Work out the finished part from the listing and answer in its coordinate system (mm). A direction names the side the tool comes from. Round coordinates to 2 decimals unless told otherwise and drop trailing zeros. Write each loop counter-clockwise with the first axis right and the second up, starting at its lowest first coordinate (ties: lowest second). Pieces come first, ordered by that corner, then holes. Notation, with made-up numbers: (55, -7.75) - (89, -7.75) arc R6 ccw to (89, -3.75) - close; hole circle Ø5 at (15.5, 87). An arc over 180 degrees is marked (long way). Write item = value, one per line. Start each with the question number.
from build123d import *

# Parameters (mm, degrees)
F0_W      = 800.1
F0_H      = 533.4
F1_DEPTH  = 1492.25
F2_W      = 647.7
F2_H      = 200.025
F2_W_2    = 311.15
F2_H_2    = 863.6
F3_DEPTH  = 12.7
F2_H_3    = 50.8
F4_DEPTH  = 533.401
F5_W      = 368.3
F5_H      = 50.8
F6_DEPTH  = 800.101
F7_W      = 596.9
F7_H      = 317.5
F8_DEPTH  = 1371.6
F9_R      = 19.05
F10_DEPTH = 12.7


with BuildPart() as f1:
    # F0 (on Top) → F1 (new body)
    with BuildSketch(Plane.XY):
        Rectangle(F0_W, F0_H)
    extrude(amount=F1_DEPTH)

    # F2 (on face) → F3 (cut)
    with BuildSketch(Plane.XZ.offset(266.7)):
        Polygon((-400.05, 0), (-323.85, 0), (-323.85, 50.8), (323.85, 50.8), (323.85, 0), (400.05, 0), (400.05, 1466.85), (-400.05, 1466.85), align=None)
        with Locations((0, 201.6125)):
            Rectangle(F2_W, F2_H, mode=Mode.SUBTRACT)
        with Locations((0, 427.0375)):
            Rectangle(F2_W, F2_H, mode=Mode.SUBTRACT)
        with Locations((-168.275, 984.25)):
            Rectangle(F2_W_2, F2_H_2, mode=Mode.SUBTRACT)
        with Locations((168.275, 984.25)):
            Rectangle(F2_W_2, F2_H_2, mode=Mode.SUBTRACT)
    extrude(amount=-F3_DEPTH, mode=Mode.SUBTRACT)

    # F2 (on face) → F4 (cut, through all)
    with BuildSketch(Plane.XZ.offset(266.7)):
        with Locations((0, 25.4)):
            Rectangle(F2_W, F2_H_3)
    extrude(amount=-F4_DEPTH, mode=Mode.SUBTRACT)

    # F5 (on face) → F6 (cut, through all)
    with BuildSketch(Plane.YZ.offset(400.05)):
        with Locations((6.35, 25.4)):
            Rectangle(F5_W, F5_H)
    extrude(amount=-F6_DEPTH, mode=Mode.SUBTRACT)

    # F7 (on face) → F8 (cut)
    with BuildSketch(Plane(origin=(0, 0, 50.8), x_dir=(1, 0, 0), z_dir=(0, 0, -1))):
        with Locations((0, -6.35)):
            Rectangle(F7_W, F7_H)
    extrude(amount=-F8_DEPTH, mode=Mode.SUBTRACT)

    # F9 (on face) → F10 (join)
    with BuildSketch(Plane.XZ.offset(266.7)):
        with Locations((-88.9, 984.25)):
            Circle(F9_R)
        with Locations((88.9, 984.25)):
            Circle(F9_R)
        with Locations((168.275, 427.0375)):
            Circle(F9_R)
        with Locations((-168.275, 427.0375)):
            Circle(F9_R)
        with Locations((-168.275, 201.6125)):
            Circle(F9_R)
        with Locations((168.275, 201.6125)):
            Circle(F9_R)
    extrude(amount=F10_DEPTH)


solid = f1.part
1. Each of these flat-tipped pins is pushed along its axis until it touches: pin 1 (10 mm diameter, centred on x = -71, y = -263, fed in from -Z); pin 2 (6.5 mm diameter, centred on y = -258.5, z = 889, fed in from +X); pin 3 (12 mm diameter, centred on x = -231.5, y = -44.5, fed in from -Z). Where does it stop, or does it pass through?
2. Find section C-C on y = 98. Give the vertices of the cut face in (x, z), plus the area to 3 significant figures.
3. Find section A-A on z = 1269. Give the vertices of the cut face in (x, y).
4. Which of the six approach directions +Z, -Z, +X, -X, +Y, -Y give full straight-line access (tool end or side, diameter ignored) to faces 5 (the face through (164.15, -272.96, 408.44)), 6 (the face through (-361, 190.5, 25)), 7 (the face through (89, -279.4, 985))?
5. Consider line 1 (Z direction, x = -57, y = -256) (3 decimals); line 2 (Y direction, x = -235, z = 538); line 3 (X direction, y = 136, z = 1265.5). Determine where each line is inside the solid, lowest interval first.
6. Find section B-B on x = -249. Give the vertices of the cut face in (y, z) (3 decimals), plus the area to 3 significant figures.
7. Find section D-D on z = 273.5. Give the vertices of the cut face in (x, y), plus the area to 3 significant figures.
8. For a pull along Y with two mould halves and no side action, classify faces 1 (the face through (-169, -279.4, 202)), 2 (the face through (-298.45, 9, 727)), 3 (the face through (-4, 165.1, 727)), 4 (the face through (-362, 229, 0)) as released by +Y, released by -Y, zero draft, split by the parting line, or undercut.
Answer key:
q1.pin_1 = 101.6
q1.pin_2 = 323.85
q1.pin_3 = 1422.4
q2.outline = (-400.05, 50.8) - (-298.45, 50.8) - (-298.45, 1422.4) - (298.45, 1422.4) - (298.45, 50.8) - (400.05, 50.8) - (400.05, 1492.25) - (-400.05, 1492.25) - close
q2.area = 335,000 mm²
q3.outline = (-400.05, -254) - (-323.85, -254) - (-323.85, -266.7) - (-12.7, -266.7) - (-12.7, -254) - (12.7, -254) - (12.7, -266.7) - (323.85, -266.7) - (323.85, -254) - (400.05, -254) - (400.05, 266.7) - (-400.05, 266.7) - close; hole (-298.45, -152.4) - (298.45, -152.4) - (298.45, 165.1) - (-298.45, 165.1) - close
q4.face_5 = -Y
q4.face_6 = -Z, +X, -X
q4.face_7 = +Z, -Z, +X, -X, -Y
q5.line_1 = 101.6 to 301.625, 327.025 to 527.05, 552.45 to 1416.05, 1466.85 to 1492.25
q5.line_2 = -254 to -152.4, 165.1 to 266.7
q5.line_3 = -400.05 to -298.45, 298.45 to 400.05
q6.outline = (-266.7, 101.6) - (-254, 101.6) - (-254, 50.8) - (-152.4, 50.8) - (-152.4, 1422.4) - (165.1, 1422.4) - (165.1, 50.8) - (266.7, 50.8) - (266.7, 1492.25) - (-266.7, 1492.25) - (-266.7, 1466.85) - (-254, 1466.85) - (-254, 1416.05) - (-266.7, 1416.05) - (-266.7, 552.45) - (-254, 552.45) - (-254, 527.05) - (-266.7, 527.05) - (-266.7, 327.025) - (-254, 327.025) - (-254, 301.625) - (-266.7, 301.625) - close
q6.area = 331,000 mm²
q7.outline = (-400.05, -254) - (-323.85, -254) - (-323.85, -266.7) - (323.85, -266.7) - (323.85, -254) - (400.05, -254) - (400.05, 266.7) - (-400.05, 266.7) - close; hole (-298.45, -152.4) - (298.45, -152.4) - (298.45, 165.1) - (-298.45, 165.1) - close
q7.area = 235,000 mm²
q8.face_1 = released by -Y
q8.face_2 = undercut
q8.face_3 = undercut
q8.face_4 = zero draft
